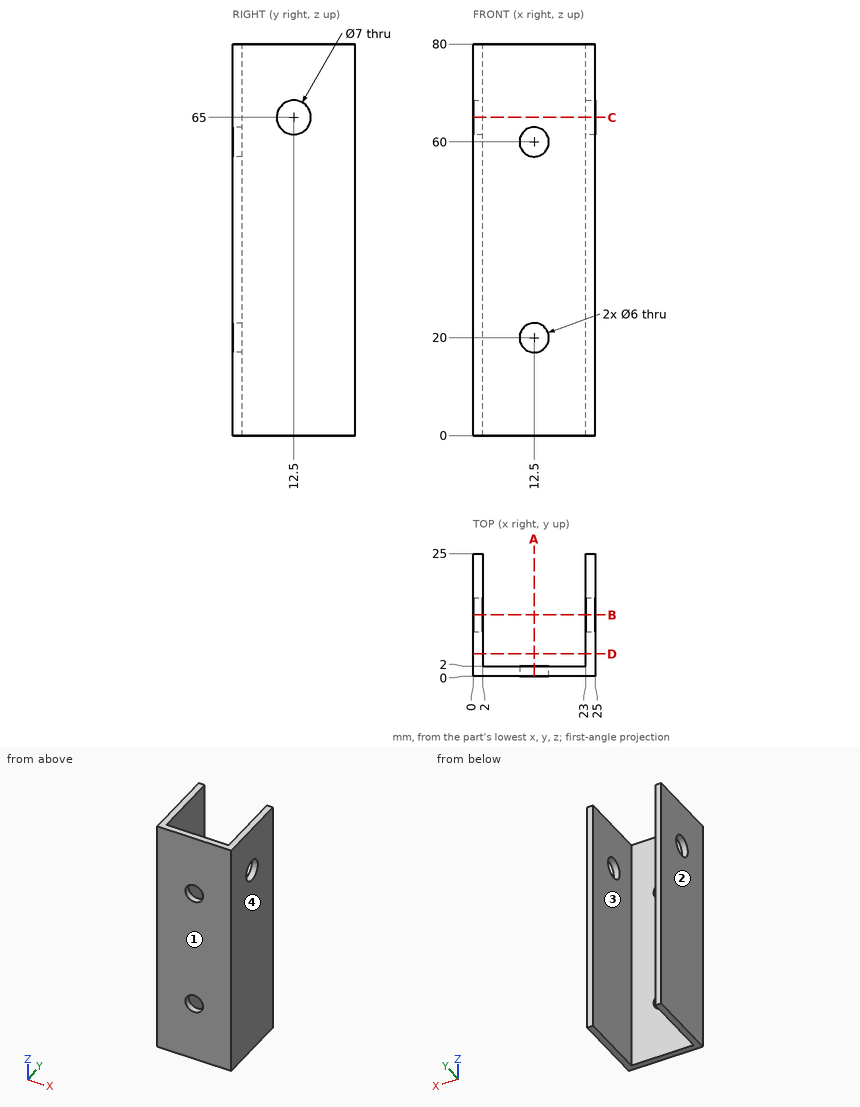
Verification items for this drawing (mm, ordinates from the low corner). Coordinates: 2 decimals unless noted, no trailing zeros. Order: outer loops, then holes, each group sorted by start corner. A loop starts at its lowest first (then second) coordinate and runs counter-clockwise, first axis right, second up. Notation, with made-up numbers: M 51.5,30 L 103.5,30 A17 cw 103.5,46 Z; hole C 81,65.25 d5. An arc over 180 degrees is marked long. One line per item, written item: value. Start each with the question number.
Item 1: Depth check by flat-ended pin: P1, Ø4, axis at y = 13, z = 62, coming from the -X side; P2, Ø7, axis at x = 12.5, z = 60, coming from the +Y side. Enter the tip coordinate at first touch or a pass-through.
Item 2: Sectioned sample at D-D on y = 4.5. Record the cut outline in (x, z).
Item 3: Sectioned sample at A-A on x = 12.5. Record the cut outline in (y, z).
Item 4: Sectioned sample at B-B on y = 12.5. Record the cut outline in (x, z), then the cut area to 3 significant figures.
Item 5: Thickness scan on probe 1 along Z at (x, y) = (12.5, 1.25); probe 2 along X at (y, z) = (5, 44.5); probe 3 along Y at (x, z) = (1.1, 65). Record the ranges inside material, lowest first.
Item 6: Sectioned sample at C-C on z = 65. Record the cut outline in (x, y), then the cut area to 3 significant figures.
Item 7: Mould release check, pull along X, two halves, no side actions. Record for the marked faces 1, 2, 3 and 4: pulls with the +X half, pulls with the -X half, needs draft (parallel to the pull), parting line crosses it, or undercut.
Calculated:
1. P1: x = 0
1. P2: y = 2
2. outline: M 0,0 L 2,0 L 2,80 L 0,80 Z; M 23,0 L 25,0 L 25,80 L 23,80 Z
3. outline: M 0,0 L 2,0 L 2,17 L 0,17 Z; M 0,23 L 2,23 L 2,57 L 0,57 Z; M 0,63 L 2,63 L 2,80 L 0,80 Z
4. outline: M 0,0 L 2,0 L 2,61.5 L 0,61.5 Z; M 0,68.5 L 2,68.5 L 2,80 L 0,80 Z; M 23,0 L 25,0 L 25,61.5 L 23,61.5 Z; M 23,68.5 L 25,68.5 L 25,80 L 23,80 Z
4. area: 292 mm^2
5. probe 1: 0 to 17, 23 to 57, 63 to 80
5. probe 2: 0 to 2, 23 to 25
5. probe 3: 0 to 9, 16 to 25
6. outline: M 0,0 L 25,0 L 25,9 L 23,9 L 23,2 L 2,2 L 2,9 L 0,9 Z; M 0,16 L 2,16 L 2,25 L 0,25 Z; M 23,16 L 25,16 L 25,25 L 23,25 Z
6. area: 114 mm^2
7. face 1: needs draft
7. face 2: pulls with the -X half
7. face 3: undercut
7. face 4: pulls with the +X half
